Autodesk Inventor part; units mm, degrees
ref_plane "YZ Plane" through (0, 0, 0) normal (1, 0, 0) x (0, 1, 0)
ref_plane "XZ Plane" through (0, 0, 0) normal (0, 1, 0) x (-1, 0, 0)
ref_plane "XY Plane" through (0, 0, 0) normal (0, 0, 1) x (1, 0, 0)
sketch "Skizze1" plane through (0, 0, 0) normal (0, 1, 0) x (-1, 0, 0)
  line L0 (37.9316, -16.2735) -> (-2.0684, -16.2735)
  line L1 (-2.0684, -16.2735) -> (-2.0684, -86.2735)
  line L2 (-2.0684, -86.2735) -> (37.9316, -86.2735)
  line L3 (37.9316, -86.2735) -> (37.9316, -16.2735)
  point P0 (0, 0)
  dimension "d0" = 70
  dimension "d1" = 40
extrude "Extrusion1" add sketch "Skizze1" along normal blind 3
fillet "Rundung1" radius 1 4 edges at (-37.9316, 1.5, -16.2735) (-37.9316, 1.5, -86.2735) (2.0684, 1.5, -86.2735) (2.0684, 1.5, -16.2735)
sketch "Skizze2" plane through (2.0684, 0, -17.2735) normal (1, 0, 0) x (0, 0, -1)
  circle A0 centre (1.5, 1.5) radius 1.5
  circle A1 centre (66.5, 1.5) radius 1.5
  line L0 (0, 3) -> (68, 3)
  line L1 (0, 0) -> (0, 3)
  line L2 (68, 3) -> (68, 0)
  point P0 (-17.2735, 0)
  dimension "d5" = 3
  dimension "d6" = 3
  dimension "d7" = 1.5
  dimension "d8" = 1.5
  dimension "d9" = 1.5
  dimension "d10" = 1.5
extrude "Extrusion2" add sketch "Skizze2" along normal blind 50 contours A0 | A1
sketch "Skizze3" plane through (52.0684, 1.5, -18.7735) normal (1, 0, 0) x (0, 0, -1)
  line L0 (-2.5, 1.5) -> (67.5, 1.5)
  line L1 (67.5, 1.5) -> (67.5, -1.5)
  line L2 (67.5, -1.5) -> (-2.5, -1.5)
  line L3 (-2.5, -1.5) -> (-2.5, 1.5)
  circle A0 centre (0, 0) radius 1.5
  circle A1 centre (65, 0) radius 1.5
  line L4 (-2.5, 20) -> (1.5, 20)
  line L5 (1.5, 20) -> (1.5, -20)
  line L6 (1.5, -20) -> (-2.5, -20)
  line L7 (-2.5, -20) -> (-2.5, 20)
  line L8 (67.5, 20) -> (63.5, 20)
  line L9 (63.5, 20) -> (63.5, -20)
  line L10 (63.5, -20) -> (67.5, -20)
  line L11 (67.5, -20) -> (67.5, 20)
  point P0 (-18.7735, -1.5)
  dimension "d13" = 1.5
  dimension "d14" = 1.5
  dimension "d16" = 2.5
  dimension "d17" = 2.5
  dimension "d20" = 40
  dimension "d21" = 20
extrude "Extrusion4" add sketch "Skizze3" against normal blind 2
sketch "Skizze4" plane through (0, 3, 0) normal (0, 1, 0) x (1, 0, 0)
  line L0 (2.0684, 14.6832) -> (-41.6445, 14.6832)
  line L1 (-41.6445, 14.6832) -> (-41.6445, 91.2635)
  line L2 (-41.6445, 91.2635) -> (2.0684, 91.2635)
  line L3 (2.0684, 91.2635) -> (2.0684, 14.6832)
  point P0 (0, 0)
extrude "Extrusion5" cut sketch "Skizze4" against normal blind 10
properties part number "Spielstraßenschild_Teil_Unten"
Input: part model. Units: mm. Frame: model coordinates. A direction names the side the tool comes from. Give positions to 0.01 mm unless a question says otherwise; leave off trailing zeros. Loops run counter-clockwise (first coordinate to the right, second up) from the corner with the lowest first, then second, coordinate; pieces in that order, holes last. Notation, with made-up numbers: (-9.75, -32.75) - (43.25, -32.75) arc R11 cw to (43.25, -25.75) - close; hole circle Ø9 at (44, 27.5). An arc over 180 degrees is marked (long way). Use CSV: the item, a comma, the result in double quotes. Start each with the question number.
Item 1: Mould query, pull axis Z, two halves, no side actions, for faces 1 (the flat face through (51, 1, -16.273)), 2 (the flat face through (2.068, 2, -19)), 3 (the flat face through (51, 1, -86.274)), 4 (the flat face through (51, 0, -52)). Classes: pulls with the +Z half, pulls with the -Z half, needs draft (parallel to the pull), parting line crosses it, or undercut.
Item 2: Line query: line 1 (X direction, y = -3, z = -82.5); line 2 (Z direction, x = 33.5, y = 0.5); line 3 (Z direction, x = 33, y = 1). Output: solid intervals per line, ascending.
Item 3: Contact query for flat-ended pins moving along their axis: P1, Ø2, axis at x = 51, z = -38, coming from the +Y side; P2, Ø12, axis at x = 44.5, y = 13.5, coming from the +Z side; P3, Ø1.6, axis at x = 51, z = -37, coming from the -Y side; P4, Ø8, axis at y = 11, z = -25.5, coming from the -X side. Output: stop coordinate, or through.
Item 4: Section C-C on x = 16. Return loops of the section in (y, z).
Item 5: Section A-A on y = 17. Return loops of the section in (x, z), then the cut area to 3 significant figures.
Item 6: Section B-B on y = 1.5. Return loops of the section in (x, z), then the cut area to 3 significant figures.
Item 7: Section D-D on z = -73.5. Return loops of the section in (x, y), then the cut area to 3 significant figures.
Item 8: Reachability of faces 5 (the flat face through (51, 3, -51)), 6 (the cylindrical face through (25.732, 1.434, -17.275)), 7 (the flat face through (51, -9, -20.274)), 8 (the flat face through (2.068, 2, -84)), 9 (the flat face through (51, 21.5, -84)) from +Z, -Z, +X, -X, +Y, -Y: full face, straight path, thin tool, end or side. Return the list, or none.
Ans:
1,face 1,"pulls with the +Z half"
1,face 2,"needs draft"
1,face 3,"pulls with the -Z half"
1,face 4,"undercut"
2,line 1,"x = 50.07 to 52.07"
2,line 2,"z = -84.89 to -82.66, -19.89 to -17.66"
2,line 3,"z = -85.19 to -82.36, -20.19 to -17.36"
3,P1,"stops at y = 3"
3,P2,"stops at z = -16.27"
3,P3,"stops at y = 0"
3,P4,"passes through"
4,outline,"circle Ø3 at (1.5, -83.77); circle Ø3 at (1.5, -18.77)"
5,outline,"(50.07, -86.27) - (52.07, -86.27) - (52.07, -82.27) - (50.07, -82.27) - close; (50.07, -20.27) - (52.07, -20.27) - (52.07, -16.27) - (50.07, -16.27) - close"
5,area,"16.0 mm2"
6,outline,"(2.07, -85.27) - (50.07, -85.27) - (50.07, -86.27) - (52.07, -86.27) - (52.07, -16.27) - (50.07, -16.27) - (50.07, -17.27) - (2.07, -17.27) - (2.07, -20.27) - (50.07, -20.27) - (50.07, -82.27) - (2.07, -82.27) - close"
6,area,"428 mm2"
7,outline,"(50.07, 0) - (52.07, 0) - (52.07, 3) - (50.07, 3) - close"
7,area,"6.00 mm2"
8,face 5,"+X, -X, +Y"
8,face 6,"-X"
8,face 7,"+X, -X, -Y"
8,face 8,"+Z, -Z, -X, +Y, -Y"
8,face 9,"+Z, -Z, +X, -X, +Y"
